The drawing under review shows one solid part. Ordinate dimensions are in mm from its lowest x, y, z. A direction names the side the tool comes from. Coordinates: 2 decimals unless noted, no trailing zeros. Write each loop counter-clockwise with the first axis right and the second up, starting at its lowest first coordinate (ties: lowest second). Pieces come first, ordered by that corner, then holes.
Q1. For probe 1 along Y at (x, z) = (3.25, 10.25); probe 2 along Z at (x, y) = (5, 10); probe 3 along Z at (x, y) = (9.5, 7), list the stretches that pass through material, from the lowest coordinate up.
Q2. Take a section at D-D (x = 5). Give the boundary of the cut face in (y, z).
Q3. Take a section at C-C (x = 2). Give the boundary of the cut face in (y, z).
Q4. Mouldability with a two-part tool opening along Z and no side actions: class the marked faces 1, 2 and 3 as pulls with the +Z half, pulls with the -Z half, needs draft (parallel to the pull), parting line crosses it, or undercut.
Q5. Machinability: for the marked faces 4 and 5, which of the approach directions +Z, -Z, +X, -X, +Y, -Y give a long, thin tool a straight path to every point of the face, cutting with its end or side? Answer none if there is none.
Q6. Take a section at A-A (y = 10). Give the boundary of the cut face in (x, z).
Q7. Insertion check: pin 1 (1.5 mm diameter, centred on x = 2.5, z = 12.5, fed in from +Y); pin 2 (10 mm diameter, centred on y = 5, z = 10, fed in from +X); pin 3 (8 mm diameter, centred on y = 10, z = 10, fed in from +X); pin 4 (6 mm diameter, centred on x = 8, z = 7, fed in from -Y). Each pin has a flat end and moves straight along its axis. Give the tip position at first contact, or say it passes through.
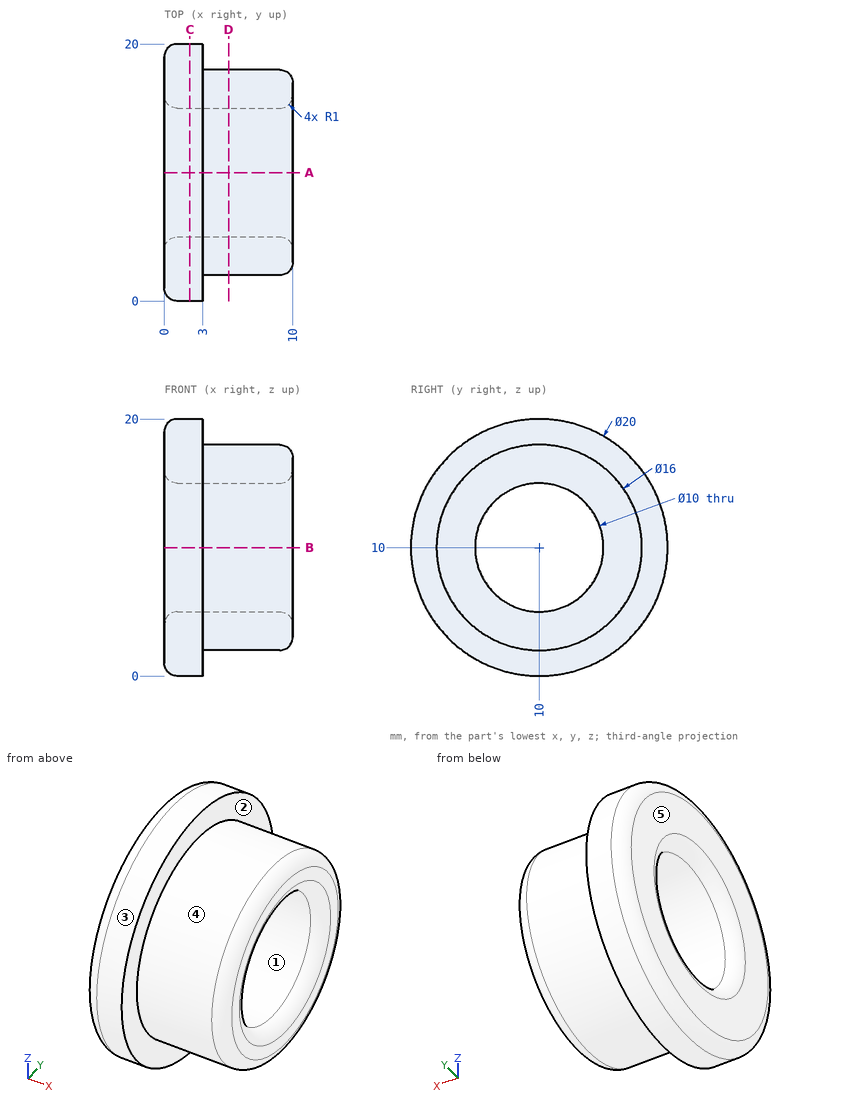
Response:
1. probe 1: y = 2 to 5.01, 14.99 to 18
1. probe 2: z = 2 to 5, 15 to 18
1. probe 3: z = 2.73 to 5.83, 14.17 to 17.27
2. outline: circle Ø16 at (10, 10); hole circle Ø10 at (10, 10)
3. outline: circle Ø20 at (10, 10); hole circle Ø10 at (10, 10)
4. face 1: undercut
4. face 2: needs draft
4. face 3: parting line crosses it
5. face 4: +X
5. face 5: +Z, -Z, -X, +Y, -Y
6. outline: (0, 1) arc R1 ccw to (1, 0) - (3, 0) - (3, 2) - (9, 2) arc R1 ccw to (10, 3) - (10, 4) arc R1 ccw to (9, 5) - (1, 5) arc R1 ccw to (0, 4) - close; (0, 16) arc R1 ccw to (1, 15) - (9, 15) arc R1 ccw to (10, 16) - (10, 17) arc R1 ccw to (9, 18) - (3, 18) - (3, 20) - (1, 20) arc R1 ccw to (0, 19) - close
7. pin 1: stops at y = 19.85
7. pin 2: stops at x = 10
7. pin 3: passes through
7. pin 4: stops at y = 2
